Check sheet for the drawn part. Datum: minimum x, y, z corner. Units: mm. A direction names the side the tool comes from. Round coordinates to 2 decimals unless told otherwise and drop trailing zeros. Order: outer loops, then holes, each group sorted by start corner. A loop starts at its lowest first (then second) coordinate and runs counter-clockwise, first axis right, second up. Notation, with made-up numbers: (-36, 85.5) -> (5, 85.5) arc R18 ccw to (5, 98.5) -> close; hole circle Ø11 at (28, -7.5). An arc over 180 degrees is marked (long way). Answer in a Markdown table with one row per item.
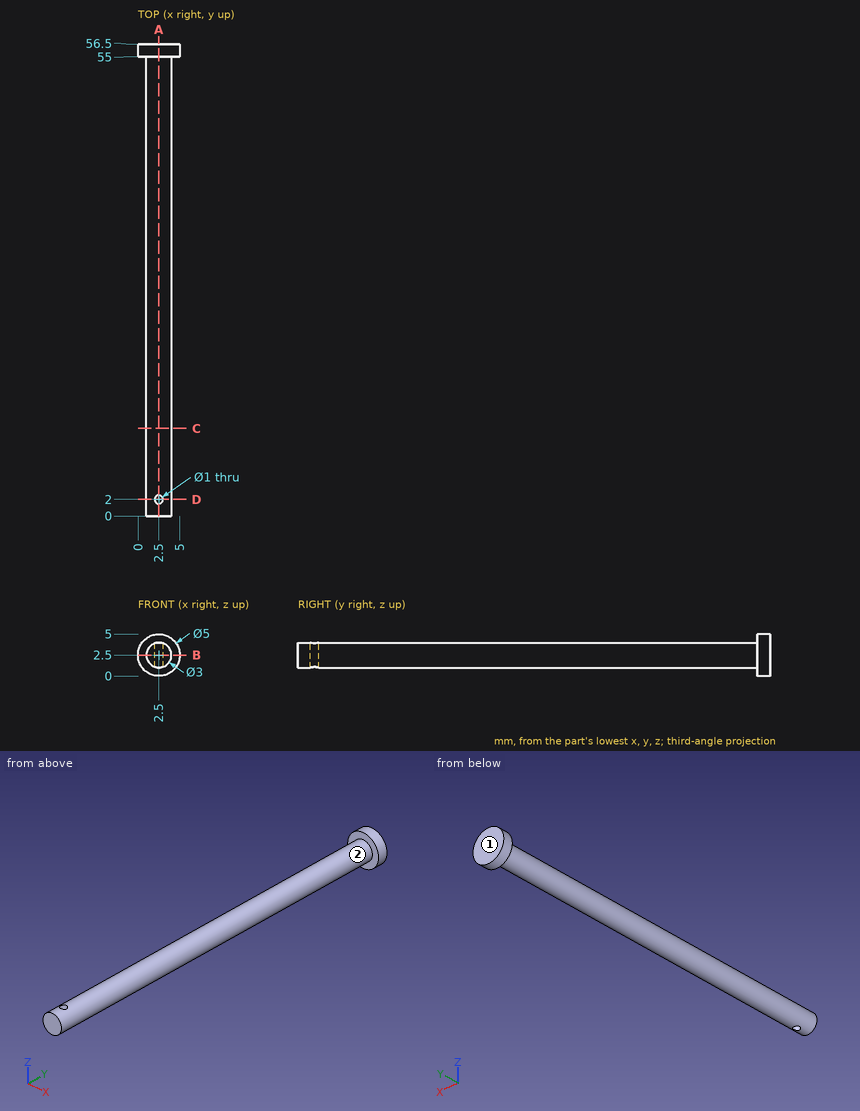
(1) Section check B-B on z = 2.5. Record the boundary of the cut face in (x, y), plus the area to 3 significant figures.
Solutions:
| item | result |
|---|---|
| outline | (0, 55) -> (1, 55) -> (1, 0) -> (4, 0) -> (4, 55) -> (5, 55) -> (5, 56.5) -> (0, 56.5) -> close; hole circle Ø1 at (2.5, 2) |
| area | 172 mm^2 |
(2) Depth check by flat-ended pin: pin 1 Ø3 at (x, y) = (4.5, 44) entering from +Z; pin 2 Ø3 at (y, z) = (26.5, 1.5) entering from -X. Enter the tip coordinate at first touch or a pass-through.
Solutions:
| item | result |
|---|---|
| pin 1 | z = 3.91 |
| pin 2 | x = 1 |
(3) Section check A-A on x = 2.5. Record the boundary of the cut face in (y, z).
Solutions:
| item | result |
|---|---|
| outline | (0, 1) -> (1.5, 1) -> (1.5, 4) -> (0, 4) -> close; (2.5, 1) -> (55, 1) -> (55, 0) -> (56.5, 0) -> (56.5, 5) -> (55, 5) -> (55, 4) -> (2.5, 4) -> close |
(4) Section check D-D on y = 2. Record the boundary of the cut face in (x, z), plus the area to 3 significant figures.
Solutions:
| item | result |
|---|---|
| outline | (2, 1.09) -> (2, 3.91) arc R1.5 ccw to start; (3, 1.09) arc R1.5 ccw to (3, 3.91) -> close |
| area | 4.13 mm^2 |
(5) Scan lines: probe 1 along Y at (x, z) = (2.6, 3.7); probe 2 along Z at (x, y) = (2.4, 32.5); probe 3 along Y at (x, z) = (3.15, 4.4). Record each from-to range of solid material in increasing order. Write a range as from..to.
Solutions:
| item | result |
|---|---|
| probe 1 | 0..1.51, 2.49..56.5 |
| probe 2 | 1..4 |
| probe 3 | 55..56.5 |
(6) Section check C-C on y = 10.5. Record the boundary of the cut face in (x, z).
Solutions:
| item | result |
|---|---|
| outline | circle Ø3 at (2.5, 2.5) |
(7) Tool access check on the marked faces 1 and 2. Record the directions out of +Z, -Z, +X, -X, +Y, -Y that give a thin tool (end or side, any length) a straight path to the whole face; none if there is none.
Solutions:
| item | result |
|---|---|
| face 1 | +Z, -Z, +X, -X, +Y |
| face 2 | -Y |
